```python
from build123d import *

# Parameters (mm, degrees)
F0_W      = 67.1
F0_H      = 138.3
F1_DEPTH  = 3.55
F2_R      = 5.08
F3_T      = -2.54
F1_FACE_W = 56.94
F1_FACE_H = 7.1
F4_DEPTH  = 7.1
F5_W      = 26.680329
F5_H      = 11.762295
F6_DEPTH  = 25
F7_R      = 13.773482
F8_DEPTH  = 12.5
F9_W      = 4.120178
F9_H      = 35.554205
F10_DEPTH = 12.5


with BuildPart() as f1:
    # F0 (on Front) → F1 (new body, symmetric)
    with BuildSketch(Plane.XZ):
        Rectangle(F0_W, F0_H)
    extrude(amount=F1_DEPTH, both=True)

    # F2
    f2_edges = [f1.edges().sort_by_distance(p)[0] for p in [
        (33.55, 0, 69.15),
        (-33.55, 0, 69.15),
        (-33.55, 0, -69.15),
        (33.55, 0, -69.15),
    ]]
    fillet(f2_edges, radius=F2_R)

    # F3
    f3_openings = [f1.faces().sort_by_distance(p)[0] for p in [
        (0, -3.55, 0),
    ]]
    offset(amount=F3_T, openings=f3_openings)

    # F1_face (on face) → F4 (cut)
    with BuildSketch(Plane(origin=(0, 0, -69.15), x_dir=(1, 0, 0), z_dir=(0, 0, -1))):
        Rectangle(F1_FACE_W, F1_FACE_H)
    extrude(amount=-F4_DEPTH, mode=Mode.SUBTRACT)

    # F5 (on Front) → F6 (cut)
    with BuildSketch(Plane.XZ):
        with Locations((-15.922133, 57.377054)):
            Rectangle(F5_W, F5_H)
    extrude(amount=-F6_DEPTH, mode=Mode.SUBTRACT)

    # F7 (on face) → F8 (cut, symmetric)
    with BuildSketch(Plane(origin=(0, 3.55, 0), x_dir=(-1, 0, 0), z_dir=(0, 1, 0))):
        with Locations((0, 23.381149)):
            Circle(F7_R)
    extrude(amount=F8_DEPTH, both=True, mode=Mode.SUBTRACT)

    # F9 (on face) → F10 (cut, symmetric)
    with BuildSketch(Plane.YZ.offset(33.55)):
        with Locations((-0.342509, 38.427914)):
            Rectangle(F9_W, F9_H)
    extrude(amount=F10_DEPTH, both=True, mode=Mode.SUBTRACT)


solid = f1.part
```
The listing builds one solid part. Answer for the finished solid, in the listing's coordinates (mm). A direction names the side the tool comes from. Round coordinates to 2 decimals unless told otherwise and drop trailing zeros. Loops run counter-clockwise (first coordinate to the right, second up) from the corner with the lowest first, then second, coordinate; pieces in that order, holes last.
1) For faces 1 (the face through (30.286, -1.302, -65.846)), 2 (the face through (-2.582, 2, 57)), 3 (the face through (28.47, 1, -67)), determine the directions among +Z, -Z, +X, -X, +Y, -Y from which every point of the face is accessible in a straight line to the end or side of a thin tool.
Outcome:
face 1: -Y
face 2: +Y, -Y
face 3: -Z, +Y, -Y
2) Given P1, Ø2, axis at y = 1, z = -66, coming from the +X side; P2, Ø2, axis at x = -9.5, y = 2, coming from the -Z side; P3, Ø1.5, axis at x = -8, z = -36, coming from the -Y side, each flat-ended and moving along its own axis, determine where each tip first touches the part or whether it passes through.
Outcome:
P1: stops at x = 33.46
P2: stops at z = -62.05
P3: stops at y = 1.01
3) Consider line 1 (X direction, y = -1.75, z = -27.5); line 2 (Z direction, x = 0, y = 1.85); line 3 (Z direction, x = -24, y = 3). Determine where each line is inside the solid, lowest interval first.
Outcome:
line 1: x = -33.55 to -31.01, 31.01 to 33.55
line 2: z = -62.05 to 9.61, 37.15 to 69.15
line 3: z = -62.05 to 51.5, 63.26 to 69.15
4) A cutting plane is placed at B-B on z = -29. Determine the outline of the cut face in (x, y), plus the area to 3 significant figures.
Outcome:
outline: (-33.55, -3.55) - (-31.01, -3.55) - (-31.01, 1.01) - (31.01, 1.01) - (31.01, -3.55) - (33.55, -3.55) - (33.55, 3.55) - (-33.55, 3.55) - close
area: 194 mm2
5) For a pull along X with two mould halves and no side action, classify faces 4 (the face through (30.6, 1.2, 56.205)), 5 (the face through (-33.55, 0, -1)), 6 (the face through (33.55, 0, -15)), 7 (the face through (-16, 2, 51.496)) as released by +X, released by -X, zero draft, split by the parting line, or undercut.
Outcome:
face 4: zero draft
face 5: released by -X
face 6: released by +X
face 7: undercut
6) A cutting plane is placed at A-A on x = 0. Determine the outline of the cut face in (y, z), plus the area to 3 significant figures.
Outcome:
outline: (-3.55, 66.61) - (1.01, 66.61) - (1.01, 37.15) - (3.55, 37.15) - (3.55, 69.15) - (-3.55, 69.15) - close; (1.01, -62.05) - (3.55, -62.05) - (3.55, 9.61) - (1.01, 9.61) - close
area: 275 mm2
7) A cutting plane is placed at D-D on x = -26. Determine the outline of the cut face in (y, z).
Outcome:
outline: (-3.55, 66.61) - (1.01, 66.61) - (1.01, 63.26) - (3.55, 63.26) - (3.55, 69.15) - (-3.55, 69.15) - close; (1.01, -62.05) - (3.55, -62.05) - (3.55, 51.5) - (1.01, 51.5) - close
8) A cutting plane is placed at C-C on x = 24.5. Determine the outline of the cut face in (y, z).
Outcome:
outline: (-3.55, 66.61) - (1.01, 66.61) - (1.01, 56.21) - (1.72, 56.21) - (1.72, 20.65) - (1.01, 20.65) - (1.01, -62.05) - (3.55, -62.05) - (3.55, 69.15) - (-3.55, 69.15) - close
